```python
from build123d import *

# Parameters (mm, degrees)
SKETCH1_W                                 = 935.736
SKETCH1_H                                 = 60.325
BASE_FLANGE1_DEPTH                        = 2.05232
EDGE_FLANGE1_DEPTH                        = 910.336
EDGE_FLANGE1_BEND_DEPTH                   = 910.336
EDGE_FLANGE2_STRIP_W                      = 13.28928
EDGE_FLANGE2_STRIP_H                      = 2.05232
EDGE_FLANGE2_STRIP_CUT_DEPTH              = 60.325
EDGE_FLANGE2_STRIP_2_W                    = 13.28928
EDGE_FLANGE2_STRIP_2_H                    = 2.05232
EDGE_FLANGE2_STRIP_CUT_2_DEPTH            = 60.325
EDGE_FLANGE2_DEPTH                        = 60.325
EDGE_FLANGE2_BEND_DEPTH                   = 60.325
HOLE_FOR_1_4_SELF_CLINCHING_NUTS_S_SS_C_D = 8.7376
BREAK_CORNER1_DEPTH                       = 935.736
BREAK_CORNER1_START                       = -64.91732
BREAK_CORNER1_2_DEPTH                     = 69.50964


# Read off the part's stored shape, not the designer's step: Break-Corner1
# Sheet-metal steps are written as plain solids
with BuildPart() as part:
    # Sketch1 → Base-Flange1 (new body)
    with BuildSketch(Plane(origin=(0, 0, 0), x_dir=(1, 0, 0), z_dir=(0, 1, 0))):
        with Locations((467.868, 30.1625)):
            Rectangle(SKETCH1_W, SKETCH1_H)
    extrude(amount=-BASE_FLANGE1_DEPTH)

    # Edge-Flange1 section (across the edge) → Edge-Flange1 (add)
    with BuildSketch(Plane(origin=(923.036, 0, -62.865), x_dir=(0, 0, 1), z_dir=(-1, 0, 0))):
        with BuildLine():
            Line((-2.05232, 2.54), (-2.05232, 31.75))
            Line((-2.05232, 31.75), (0, 31.75))
            Line((0, 31.75), (0, 2.54))
            ThreePointArc((0, 2.54), (0.743948776, 0.743948776), (2.54, 0))
            Line((2.54, 0), (2.54, -2.05232))
            ThreePointArc((2.54, -2.05232), (-0.707260613, -0.707260613), (-2.05232, 2.54))
        make_face()
    extrude(amount=EDGE_FLANGE1_DEPTH)

    # Edge-Flange1 section 2 (across the edge) → Edge-Flange1 bend (add)
    with BuildSketch(Plane(origin=(12.7, 0, 2.54), x_dir=(0, 0, -1), z_dir=(1, 0, 0))):
        with BuildLine():
            Line((-2.05232, 2.54), (-2.05232, 31.75))
            Line((-2.05232, 31.75), (0, 31.75))
            Line((0, 31.75), (0, 2.54))
            ThreePointArc((0, 2.54), (0.743948776, 0.743948776), (2.54, 0))
            Line((2.54, 0), (2.54, -2.05232))
            ThreePointArc((2.54, -2.05232), (-0.707260613, -0.707260613), (-2.05232, 2.54))
        make_face()
    extrude(amount=EDGE_FLANGE1_BEND_DEPTH)

    # Edge-Flange2 strip (across the edge) → Edge-Flange2 strip cut (cut)
    with BuildSketch(Plane.XY.offset(-60.325)):
        with Locations((-2.05232, -1.02616)):
            Rectangle(EDGE_FLANGE2_STRIP_W, EDGE_FLANGE2_STRIP_H)
    extrude(amount=EDGE_FLANGE2_STRIP_CUT_DEPTH, mode=Mode.SUBTRACT)

    # Edge-Flange2 strip 2 (across the edge) → Edge-Flange2 strip cut 2 (cut)
    with BuildSketch(Plane(origin=(935.736, 0, 0), x_dir=(-1, 0, 0), z_dir=(0, 0, -1))):
        with Locations((-2.05232, -1.02616)):
            Rectangle(EDGE_FLANGE2_STRIP_2_W, EDGE_FLANGE2_STRIP_2_H)
    extrude(amount=EDGE_FLANGE2_STRIP_CUT_2_DEPTH, mode=Mode.SUBTRACT)

    # Edge-Flange2 section (across the edge) → Edge-Flange2 (add)
    with BuildSketch(Plane.XY.offset(-60.325)):
        with BuildLine():
            Line((0, 2.54), (0, 61.44768))
            Line((0, 61.44768), (2.05232, 61.44768))
            Line((2.05232, 61.44768), (2.05232, 2.54))
            ThreePointArc((2.05232, 2.54), (2.796268776, 0.743948776), (4.59232, 0))
            Line((4.59232, 0), (4.59232, -2.05232))
            ThreePointArc((4.59232, -2.05232), (1.345059387, -0.707260613), (0, 2.54))
        make_face()
    extrude(amount=EDGE_FLANGE2_DEPTH)

    # Edge-Flange2 section 2 (across the edge) → Edge-Flange2 bend (add)
    with BuildSketch(Plane(origin=(935.736, 0, 0), x_dir=(-1, 0, 0), z_dir=(0, 0, -1))):
        with BuildLine():
            Line((0, 2.54), (0, 61.44768))
            Line((0, 61.44768), (2.05232, 61.44768))
            Line((2.05232, 61.44768), (2.05232, 2.54))
            ThreePointArc((2.05232, 2.54), (2.796268776, 0.743948776), (4.59232, 0))
            Line((4.59232, 0), (4.59232, -2.05232))
            ThreePointArc((4.59232, -2.05232), (1.345059387, -0.707260613), (0, 2.54))
        make_face()
    extrude(amount=EDGE_FLANGE2_BEND_DEPTH)

    # Hole for 1/4 Self-clinching Nuts (S,SS,CLS,CLSS)1 (through all)
    with Locations(Plane.ZY):
        with Locations((-47.625, 29.69768), (-12.7, 29.69768)):
            Hole(HOLE_FOR_1_4_SELF_CLINCHING_NUTS_S_SS_C_D / 2)

    # Break-Corner1 outline → Break-Corner1 (cut)
    with BuildSketch(Plane.YZ):
        with BuildLine():
            ThreePointArc((55.09768, 0), (59.587808061, -1.859871939), (61.44768, -6.35))
            Line((61.44768, -6.35), (61.44768, 0))
            Line((61.44768, 0), (55.09768, 0))
        make_face()
        with BuildLine():
            Line((61.44768, -60.325), (61.44768, -53.975))
            ThreePointArc((61.44768, -53.975), (59.587808061, -58.465128061), (55.09768, -60.325))
            Line((55.09768, -60.325), (61.44768, -60.325))
        make_face()
    extrude(amount=BREAK_CORNER1_DEPTH, mode=Mode.SUBTRACT)

    # Break-Corner1 2 outline → Break-Corner1 2 (cut)
    with BuildSketch(Plane.XY.offset(BREAK_CORNER1_START)):
        with BuildLine():
            Line((12.7, 31.75), (12.7, 25.4))
            ThreePointArc((12.7, 25.4), (14.559871939, 29.890128061), (19.05, 31.75))
            Line((19.05, 31.75), (12.7, 31.75))
        make_face()
        with BuildLine():
            Line((923.036, 31.75), (916.686, 31.75))
            ThreePointArc((916.686, 31.75), (921.176128061, 29.890128061), (923.036, 25.4))
            Line((923.036, 25.4), (923.036, 31.75))
        make_face()
    extrude(amount=BREAK_CORNER1_2_DEPTH, mode=Mode.SUBTRACT)


solid = part.part
```
Geometry: final body of the model. Coordinates: model frame, mm. A direction names the side the tool comes from. Coordinates: 2 decimals unless noted, no trailing zeros. Order: outer loops, then holes, each group sorted by start corner. A loop starts at its lowest first (then second) coordinate and runs counter-clockwise, first axis right, second up.
Item 1: Draft query along Z for faces 6 (the face through (461, -2.052, -31)), 7 (the face through (461, 17, 2.54)), 8 (the face through (474, 17, -64.917)), 9 (the face through (461, 17, 4.592)). Return one class per face: released by +Z, released by -Z, zero draft, split by the parting line, or undercut.
Answer:
face 6: zero draft
face 7: undercut
face 8: released by -Z
face 9: released by +Z
Item 2: Material intervals for line 1 along X through (y, z) = (31, -19.5); line 2 along Z through (x, y) = (64.5, 19) (3 decimals); line 3 along Y through (x, z) = (375, -40.5), sorted ascending.
Answer:
line 1: x = 0 to 2.05, 933.68 to 935.74
line 2: z = -64.917 to -62.865, 2.54 to 4.592
line 3: y = -2.05 to 0
Item 3: Section query C-C (x = 765). Output: boundary loops of the cut face in (y, z) (3 decimals).
Answer:
outline: (-2.052, -60.325) arc R4.592 ccw to (2.54, -64.917) - (31.75, -64.917) - (31.75, -62.865) - (2.54, -62.865) arc R2.54 cw to (0, -60.325) - (0, 0) arc R2.54 cw to (2.54, 2.54) - (31.75, 2.54) - (31.75, 4.592) - (2.54, 4.592) arc R4.592 ccw to (-2.052, 0) - close
Item 4: Access query for faces 1 (the face through (0, 32, -31)), 2 (the face through (935.736, 32, -30)), 3 (the face through (461, 0, -31)), 4 (the face through (2.052, 32, -31)), 5 (the face through (474, 17, -62.865)). Directions: +Z, -Z, +X, -X, +Y, -Y. A direction counts if a zero-diameter tool reaches every point of the face in a straight line with its end or side. Return the directions, or none.
Answer:
face 1: +Z, -Z, -X, +Y, -Y
face 2: +Z, -Z, +X, +Y, -Y
face 3: +Y
face 4: +Z, -Z, +Y
face 5: +X, -X, +Y
Item 5: Section query A-A (y = 47). Output: boundary loops of the cut face in (x, z) (3 decimals), then the cut area to 3 significant figures.
Answer:
outline: (0, -60.325) - (2.052, -60.325) - (2.052, 0) - (0, 0) - close; (933.684, -60.325) - (935.736, -60.325) - (935.736, 0) - (933.684, 0) - close
area: 248 mm2
Item 6: Section query B-B (z = -29.5). Output: boundary loops of the cut face in (x, y).
Answer:
outline: (0, 2.54) arc R4.59 ccw to (4.59, -2.05) - (931.14, -2.05) arc R4.59 ccw to (935.74, 2.54) - (935.74, 61.45) - (933.68, 61.45) - (933.68, 2.54) arc R2.54 cw to (931.14, 0) - (4.59, 0) arc R2.54 cw to (2.05, 2.54) - (2.05, 61.45) - (0, 61.45) - close
Item 7: Contact query for flat-ended pins moving along their axis: P1, Ø14, axis at x = 6, y = 33.5, coming from the -Z side (3 decimals); P2, Ø5, axis at y = 29.7, z = -47.62, coming from the -X side; P3, Ø1.5, axis at x = 259, z = -36.5, coming from the +Y side; P4, Ø5, axis at y = 15, z = -62, coming from the +X side. Output: stop coordinate, or through.
Answer:
P1: stops at z = -60.325
P2: passes through
P3: stops at y = 0
P4: stops at x = 935.74
